CAD build for the part. Positions are in the model's coordinates, mm. A direction names the side the tool comes from. Give positions to 0.01 mm unless a question says otherwise; leave off trailing zeros. Order: outer loops, then holes, each group sorted by start corner. A loop starts at its lowest first (then second) coordinate and runs counter-clockwise, first axis right, second up.
Item 1: Which spindle directions (+Z, -Z, +X, -X, +Y, -Y) get a long thin tool onto all of the face, cutting with end or side? Do faces 4 (the flat face through (-12.7, 3, -37)), 5 (the flat face through (112, -16.51, 0)), 6 (the cylindrical face through (95.23, -2.28, 2.59)). Say none if no direction does.
Item 2: Flat gauge pins, fed straight in: P1, Ø7.5, axis at x = 0, z = -25, coming from the +Y side; P2, Ø25, axis at x = 0, z = 0, coming from the +Y side; P3, Ø8.5, axis at y = -6.35, z = 0, coming from the -X side. Where does each tip first touch, or does it go through?
Item 3: Wall check: L1, parallel to Y at x = 98, z = 32; L2, parallel to Y at x = -1, z = -15; L3, parallel to X at y = 3.9, z = -25. Give the ranges that are in metal, low to high.
Item 4: Band-saw the part on D-D on y = -14.25. Give the cut face in (x, z), plus the area to 3 significant figures.
Item 5: Band-saw the part on B-B on z = 25. Give the cut face in (x, y).
Item 6: Band-saw the part on C-C on x = 28.5. Give the cut face in (y, z), plus the area to 3 significant figures.
Item 7: Band-saw the part on A-A on z = 10. Give the cut face in (x, y), plus the area to 3 significant figures.
Item 8: Two-plate mould, pull along X, no slides. Class faces 1 (the flat face through (93.98, -5, 7)), 2 (the flat face through (-12.7, 3, 37)), 3 (the flat face through (98, -13, 16.554)): released by +X, released by -X, zero draft, split by the parting line, or undercut.
```python
from build123d import *

# Parameters (mm, degrees)
SKETCH1_R            = 30.5
BOSS_EXTRUDE1_DEPTH  = 5
SKETCH2_R            = 15.75
CUT_EXTRUDE1_DEPTH   = 2.5
SKETCH3_R            = 15.75
BOSS_EXTRUDE2_DEPTH  = 2.5
SKETCH4_R            = 3.25
CUT_EXTRUDE2_DEPTH   = 5.08
SKETCH5_R            = 3.25
CUT_EXTRUDE3_DEPTH   = 5.08
SKETCH6_R            = 3.25
CUT_EXTRUDE4_DEPTH   = 5.08
BOSS_EXTRUDE3_DEPTH  = 5.08
BOSS_EXTRUDE4_DEPTH  = 5.08
SKETCH9_W            = 17.526
SKETCH9_H            = 5.08
BOSS_EXTRUDE5_DEPTH  = 106.68
SKETCH10_W           = 17.526
SKETCH10_H           = 5.08
BOSS_EXTRUDE6_DEPTH  = 106.68
SKETCH11_W           = 25.4
SKETCH11_H           = 5.08
BOSS_EXTRUDE8_DEPTH  = 63.5
SKETCH14_W           = 93.56025604
SKETCH14_H           = 5.08
CUT_EXTRUDE6_DEPTH   = 17.78
SKETCH15_W           = 7.62
SKETCH15_H           = 33.10825604
BOSS_EXTRUDE10_DEPTH = 20.32
SKETCH16_W           = 33.10825604
SKETCH16_H           = 3.81
BOSS_EXTRUDE11_DEPTH = 20.32
CUT_EXTRUDE7_DEPTH   = 7.62
SKETCH18_R           = 4.826
CUT_EXTRUDE8_DEPTH   = 2.54


with BuildPart() as part:
    # Sketch1 → Boss-Extrude1 (new body)
    with BuildSketch(Plane(origin=(0, 0, 0), x_dir=(1, 0, 0), z_dir=(0, 1, 0))):
        with Locations(Location((0, 0, 0), (0, 0, 270))):
            Circle(SKETCH1_R)
    extrude(amount=BOSS_EXTRUDE1_DEPTH)

    # Sketch2 → Cut-Extrude1 (cut)
    with BuildSketch(Plane(origin=(0, 5, 0), x_dir=(1, 0, 0), z_dir=(0, 1, 0))):
        with Locations(Location((0, 0, 0), (0, 0, 270))):
            Circle(SKETCH2_R)
    extrude(amount=-CUT_EXTRUDE1_DEPTH, mode=Mode.SUBTRACT)

    # Sketch3 → Boss-Extrude2 (add)
    with BuildSketch(Plane.XZ):
        with Locations(Location((0, 0, 0), (0, 0, 90))):
            Circle(SKETCH3_R)
    extrude(amount=BOSS_EXTRUDE2_DEPTH)

    # Sketch4 → Cut-Extrude2 (cut)
    with BuildSketch(Plane(origin=(0, 0, 0), x_dir=(-1, 0, 0), z_dir=(0, -1, 0))):
        with Locations(Location((0, 25, 0), (0, 0, 90))):
            Circle(SKETCH4_R)
    extrude(amount=-CUT_EXTRUDE2_DEPTH, mode=Mode.SUBTRACT)

    # Sketch5 → Cut-Extrude3 (cut)
    with BuildSketch(Plane.XZ):
        with Locations(Location((0, 25, 0), (0, 0, 270))):
            Circle(SKETCH5_R)
    extrude(amount=-CUT_EXTRUDE3_DEPTH, mode=Mode.SUBTRACT)

    # Sketch6 → Cut-Extrude4 (cut)
    with BuildSketch(Plane.XZ):
        with Locations(Location((17.674476483, 17.680862, 0), (0, 0, 270))):
            Circle(SKETCH6_R)
    extrude(amount=-CUT_EXTRUDE4_DEPTH, mode=Mode.SUBTRACT)

    # Sketch7 → Boss-Extrude3 (add)
    with BuildSketch(Plane(origin=(0, 0, 0), x_dir=(-1, 0, 0), z_dir=(0, -1, 0))):
        with BuildLine():
            ThreePointArc((12.7, -27.73012802), (6.499272859, -29.79948745), (0, -30.5))
            ThreePointArc((0, -30.5), (-6.499272859, -29.79948745), (-12.7, -27.73012802))
            Line((-12.7, -27.73012802), (-12.7, -46.78012802))
            Line((-12.7, -46.78012802), (12.7, -46.78012802))
            Line((12.7, -46.78012802), (12.7, -27.73012802))
        make_face()
    extrude(amount=-BOSS_EXTRUDE3_DEPTH)

    # Sketch8 → Boss-Extrude4 (add)
    with BuildSketch(Plane.XZ):
        with BuildLine():
            ThreePointArc((0, -30.5), (-6.499272859, -29.79948745), (-12.7, -27.73012802))
            Line((-12.7, -27.73012802), (-12.7, -46.78012802))
            Line((-12.7, -46.78012802), (12.7, -46.78012802))
            Line((12.7, -46.78012802), (12.7, -27.73012802))
            ThreePointArc((12.7, -27.73012802), (6.499272859, -29.79948745), (0, -30.5))
        make_face()
    extrude(amount=-BOSS_EXTRUDE4_DEPTH)

    # Sketch9 → Boss-Extrude5 (add)
    with BuildSketch(Plane(origin=(12.7, 0, 0), x_dir=(0, 0, -1), z_dir=(1, 0, 0))):
        with Locations((38.01712802, 2.54)):
            Rectangle(SKETCH9_W, SKETCH9_H)
    extrude(amount=BOSS_EXTRUDE5_DEPTH)

    # Sketch10 → Boss-Extrude6 (add)
    with BuildSketch(Plane(origin=(12.7, 0, 0), x_dir=(0, 0, -1), z_dir=(1, 0, 0))):
        with Locations((-38.01712802, 2.54)):
            Rectangle(SKETCH10_W, SKETCH10_H)
    extrude(amount=BOSS_EXTRUDE6_DEPTH)

    # Sketch11 → Boss-Extrude8 (add)
    with BuildSketch(Plane(origin=(0, 0, 29.25412802), x_dir=(-1, 0, 0), z_dir=(0, 0, -1))):
        with Locations((-106.68, 2.54)):
            Rectangle(SKETCH11_W, SKETCH11_H)
    extrude(amount=BOSS_EXTRUDE8_DEPTH)

    # Sketch14 → Cut-Extrude6 (cut)
    with BuildSketch(Plane(origin=(119.38, 0, 0), x_dir=(0, 0, -1), z_dir=(1, 0, 0))):
        with Locations((0, 2.54)):
            Rectangle(SKETCH14_W, SKETCH14_H)
    extrude(amount=-CUT_EXTRUDE6_DEPTH, mode=Mode.SUBTRACT)

    # Sketch15 → Boss-Extrude10 (add)
    with BuildSketch(Plane.XZ):
        with Locations((97.79, 0)):
            Rectangle(SKETCH15_W, SKETCH15_H)
    extrude(amount=BOSS_EXTRUDE10_DEPTH)

    # Sketch16 → Boss-Extrude11 (add)
    with BuildSketch(Plane(origin=(101.6, 0, 0), x_dir=(0, 0, -1), z_dir=(1, 0, 0))):
        with Locations((0, -18.415)):
            Rectangle(SKETCH16_W, SKETCH16_H)
    extrude(amount=BOSS_EXTRUDE11_DEPTH)

    # Sketch17 → Cut-Extrude7 (cut)
    with BuildSketch(Plane.ZY.offset(-93.98)):
        with BuildLine():
            ThreePointArc((0, -3.048), (-3.302, -6.35), (0, -9.652))
            Line((0, -9.652), (0, -3.048))
        make_face()
        with BuildLine():
            Line((0, -3.048), (0, -9.652))
            ThreePointArc((0, -9.652), (2.334866591, -8.684866591), (3.302, -6.35))
            ThreePointArc((3.302, -6.35), (2.334866591, -4.015133409), (0, -3.048))
        make_face()
    extrude(amount=-CUT_EXTRUDE7_DEPTH, mode=Mode.SUBTRACT)

    # Sketch18 → Cut-Extrude8 (cut)
    with BuildSketch(Plane.ZY.offset(-93.98)):
        with Locations((0, -6.35)):
            Circle(SKETCH18_R)
    extrude(amount=-CUT_EXTRUDE8_DEPTH, mode=Mode.SUBTRACT)


solid = part.part
```
The answers:
1. face 4: -Z, -X, +Y, -Y
1. face 5: +Z, -Z, +X, +Y
1. face 6: none
2. P1: stops at y = 5
2. P2: stops at y = 2.5
2. P3: stops at x = -15.75
3. L1: y = 0 to 5.08
3. L2: y = -2.5 to 2.5
3. L3: x = -17.47 to -3.25, 3.25 to 17.47, 93.98 to 101.6
4. outline: (93.98, -16.55) - (101.6, -16.55) - (101.6, 16.55) - (93.98, 16.55) - close
4. area: 252 mm2
5. outline: (-17.47, 0) - (-3.25, 0) - (-3.25, 5) - (-17.47, 5) - close; (3.25, 0) - (17.47, 0) - (17.47, 5) - (3.25, 5) - close; (93.98, 0) - (101.6, 0) - (101.6, 5.08) - (93.98, 5.08) - close
6. outline: (0, -46.78) - (5.08, -46.78) - (5.08, -29.25) - (0, -29.25) - close; (0, -10.86) - (5, -10.86) - (5, 10.86) - (0, 10.86) - close; (0, 29.25) - (5.08, 29.25) - (5.08, 46.78) - (0, 46.78) - close
6. area: 287 mm2
7. outline: (-28.81, 0) - (-12.17, 0) - (-12.17, -2.5) - (12.17, -2.5) - (12.17, 0) - (28.81, 0) - (28.81, 5) - (12.17, 5) - (12.17, 2.5) - (-12.17, 2.5) - (-12.17, 5) - (-28.81, 5) - close; (93.98, -20.32) - (121.92, -20.32) - (121.92, -16.51) - (101.6, -16.51) - (101.6, 5.08) - (93.98, 5.08) - close
7. area: 559 mm2
8. face 1: undercut
8. face 2: released by -X
8. face 3: zero draft
